```python
from build123d import *

# Parameters (mm, degrees)
SKETCH1_W           = 50.8
SKETCH1_H           = 82.55
BOSS_EXTRUDE1_DEPTH = 12.7
CUT_EXTRUDE1_DEPTH  = 1.27
SKETCH3_W           = 2.998982734
SKETCH3_H           = 7.14554636
SKETCH3_W_2         = 3.079931229
BOSS_EXTRUDE2_DEPTH = 12.7


with BuildPart() as part:
    # Sketch1 → Boss-Extrude1 (new body)
    with BuildSketch(Plane(origin=(0, 0, 0), x_dir=(1, 0, 0), z_dir=(0, 1, 0))):
        Rectangle(SKETCH1_W, SKETCH1_H)
    extrude(amount=BOSS_EXTRUDE1_DEPTH)

    # Sketch2 → Cut-Extrude1 (cut)
    with BuildSketch(Plane(origin=(0, 12.7, 0), x_dir=(1, 0, 0), z_dir=(0, 1, 0))):
        Polygon((-1.861676083, 3.013416612), (-0.314881211, 3.013416612), (-0.314881211, 2.687775586), (-1.576740185, 2.687775586), (-1.576740185, 1.710852509), (-0.314881211, 1.710852509), (-0.314881211, 1.385211483), (-1.576740185, 1.385211483), (-1.576740185, -0.161583388), (-1.861676083, -0.161583388), align=None)
        with BuildLine():
            Line((3.185759815, 2.430824464), (2.936440905, 2.240019176))
            add(Edge.make_bspline(
                [(2.936440905, 2.240019176), (2.918655563, 2.261215448), (2.883324665, 2.303322222), (2.826483817, 2.36244938), (2.767245898, 2.417844296), (2.705633552, 2.469770858), (2.64053778, 2.51641321), (2.573535484, 2.560201996), (2.503505828, 2.599452015), (2.406666755, 2.647043439), (2.279986207, 2.696706022), (2.120515174, 2.73834681), (1.954044392, 2.764854591), (1.840472284, 2.767725555), (1.782704927, 2.769185842)],
                knots=[0, 0, 0, 0, 0.757959112, 1.505699292, 2.245454638, 2.979532153, 3.711538275, 4.438200793, 5.171680507, 5.909471876, 7.393775596, 8.890124382, 10.418191784, 12, 12, 12, 12], degree=3))
            add(Edge.make_bspline(
                [(1.782704927, 2.769185842), (1.750879363, 2.768819391), (1.687523605, 2.768089888), (1.593499633, 2.758465896), (1.501231365, 2.744939298), (1.410778821, 2.724868469), (1.322257137, 2.699493308), (1.235087601, 2.669171682), (1.150532271, 2.631656935), (1.06742144, 2.590193013), (0.987793156, 2.543359546), (0.912450363, 2.492275291), (0.841667849, 2.437511896), (0.775389622, 2.378864107), (0.713547926, 2.316596042), (0.656590866, 2.250044104), (0.604715529, 2.179421061), (0.556893657, 2.105658184), (0.514064963, 2.02897033), (0.478205715, 1.949073659), (0.446451069, 1.867336366), (0.421323898, 1.782834956), (0.40143523, 1.696164018), (0.387712278, 1.607090946), (0.378197736, 1.515801822), (0.377471861, 1.453926232), (0.377105969, 1.422736523)],
                knots=[0, 0, 0, 0, 1.054917814, 2.100044995, 3.131103042, 4.146048494, 5.169673617, 6.183595914, 7.203665975, 8.234915748, 9.262203917, 10.264457458, 11.251630812, 12.227803204, 13.197192746, 14.159520551, 15.12972552, 16.100847026, 17.073214652, 18.039054194, 19.002613845, 19.979014051, 20.95965708, 21.949030935, 22.966165397, 24, 24, 24, 24], degree=3))
            add(Edge.make_bspline(
                [(0.377105969, 1.422736523), (0.378250619, 1.375808826), (0.380497988, 1.283672517), (0.400498976, 1.14871632), (0.430892881, 1.019429709), (0.476445582, 0.896620852), (0.532615007, 0.778775413), (0.603590419, 0.66788731), (0.685792563, 0.562280855), (0.780384358, 0.464451896), (0.884166777, 0.375085873), (0.995516668, 0.296390703), (1.114156701, 0.230790774), (1.23877693, 0.176202594), (1.370336333, 0.134241134), (1.508598332, 0.104700822), (1.653262214, 0.085431129), (1.752113026, 0.083586284), (1.802421474, 0.082647381)],
                knots=[0, 0, 0, 0, 1.029171465, 2.020641659, 2.987623507, 3.938342917, 4.889210282, 5.84687017, 6.821220943, 7.821438502, 8.827599549, 9.822697543, 10.807740252, 11.797342354, 12.80366471, 13.83203677, 14.896651826, 16, 16, 16, 16], degree=3))
            add(Edge.make_bspline(
                [(1.802421474, 0.082647381), (1.857850341, 0.084179345), (1.966947613, 0.087194618), (2.126938608, 0.11273908), (2.280096767, 0.154157334), (2.426430328, 0.212121877), (2.565526757, 0.28747396), (2.697603727, 0.37882132), (2.822772723, 0.487032879), (2.89803953, 0.569658288), (2.936440905, 0.611814047)],
                knots=[0, 0, 0, 0, 1.028121516, 2.023589091, 2.998037872, 3.967518031, 4.937445131, 5.927275754, 6.942489185, 8, 8, 8, 8], degree=3))
            Line((2.936440905, 0.611814047), (3.185759815, 0.422916812))
            add(Edge.make_bspline(
                [(3.185759815, 0.422916812), (3.16569553, 0.397028359), (3.125663066, 0.345375458), (3.060840436, 0.27255755), (2.992553173, 0.204064603), (2.920294065, 0.140448832), (2.844894354, 0.080437281), (2.765000185, 0.025734906), (2.681661848, -0.024421825), (2.595161714, -0.070347678), (2.505591686, -0.111094038), (2.413059092, -0.145977098), (2.317962784, -0.176026105), (2.220298416, -0.200747505), (2.119863408, -0.220043417), (2.017020192, -0.232942693), (1.911546805, -0.241780001), (1.84038923, -0.242585468), (1.804329526, -0.242993645)],
                knots=[0, 0, 0, 0, 0.986787822, 1.968848986, 2.935600012, 3.899624008, 4.868462664, 5.837806735, 6.815139263, 7.798259679, 8.787526145, 9.778297419, 10.776456485, 11.791383307, 12.812564526, 13.85620153, 14.913611965, 16, 16, 16, 16], degree=3))
            add(Edge.make_bspline(
                [(1.804329526, -0.242993645), (1.770181343, -0.24275598), (1.702657538, -0.242286028), (1.602963671, -0.234673133), (1.505908837, -0.224286586), (1.411770426, -0.208647324), (1.32003472, -0.190192101), (1.231533333, -0.165453176), (1.145395392, -0.137740717), (1.061966969, -0.105169765), (0.981177098, -0.0684158), (0.903286355, -0.026876314), (0.828330563, 0.019099377), (0.755572788, 0.068497851), (0.686087837, 0.122905832), (0.619273568, 0.181567708), (0.554755321, 0.24428576), (0.5148386, 0.289511234), (0.49476923, 0.312249745)],
                knots=[0, 0, 0, 0, 1.114604814, 2.203992996, 3.262667896, 4.300477797, 5.318619304, 6.316056647, 7.298880507, 8.271930387, 9.238335007, 10.195173496, 11.151986948, 12.108099108, 13.064862484, 14.031167946, 15.010108607, 16, 16, 16, 16], degree=3))
            add(Edge.make_bspline(
                [(0.49476923, 0.312249745), (0.462624039, 0.351747823), (0.398721742, 0.430267125), (0.316964872, 0.557526551), (0.246981019, 0.69039414), (0.190397148, 0.829567933), (0.146162382, 0.974735634), (0.115518013, 1.125970422), (0.095604771, 1.283131055), (0.093327581, 1.390025856), (0.092170071, 1.444361123)],
                knots=[0, 0, 0, 0, 0.994628077, 1.977248131, 2.950237994, 3.925870899, 4.908910175, 5.911660606, 6.938484602, 8, 8, 8, 8], degree=3))
            add(Edge.make_bspline(
                [(0.092170071, 1.444361123), (0.093580854, 1.501470713), (0.096356481, 1.613830266), (0.119938381, 1.778725209), (0.157874003, 1.936705407), (0.211755467, 2.087475946), (0.280068178, 2.231829843), (0.364456606, 2.368664365), (0.463940371, 2.498854605), (0.577739236, 2.620425129), (0.702532462, 2.731585828), (0.836171672, 2.829381455), (0.978395295, 2.910768059), (1.127636489, 2.978800292), (1.285012786, 3.031092055), (1.450188413, 3.06769816), (1.622853, 3.090482973), (1.740656772, 3.09336334), (1.800513421, 3.094826868)],
                knots=[0, 0, 0, 0, 1.032925535, 2.032216505, 3.007276963, 3.968222605, 4.92396291, 5.891752235, 6.871517503, 7.883894988, 8.900124299, 9.891468569, 10.874487609, 11.85992873, 12.854644235, 13.869047385, 14.917252991, 16, 16, 16, 16], degree=3))
            add(Edge.make_bspline(
                [(1.800513421, 3.094826868), (1.836993692, 3.0943895), (1.909202714, 3.093523773), (2.016021192, 3.085081773), (2.12001816, 3.071008716), (2.221265265, 3.051853424), (2.320255067, 3.02807964), (2.416231, 2.997109512), (2.509756237, 2.961697801), (2.600240932, 2.92091405), (2.687250946, 2.875133506), (2.770759177, 2.824863619), (2.850102299, 2.77016671), (2.925838612, 2.711507972), (2.996701175, 2.647646422), (3.064701944, 2.580338603), (3.127531637, 2.507645776), (3.166314892, 2.456478444), (3.185759815, 2.430824464)],
                knots=[0, 0, 0, 0, 1.096760587, 2.17092713, 3.219439832, 4.250915756, 5.268269357, 6.278326846, 7.281116186, 8.274029601, 9.260640565, 10.235837813, 11.203064059, 12.156899882, 13.114053108, 14.069676657, 15.032185724, 16, 16, 16, 16], degree=3))
        make_face()
    extrude(amount=-CUT_EXTRUDE1_DEPTH, mode=Mode.SUBTRACT)

    # Sketch3 → Boss-Extrude2 (add)
    with BuildSketch(Plane.XY.offset(41.275)):
        with Locations((20.244451429, 6.168632911)):
            Rectangle(SKETCH3_W, SKETCH3_H)
        with Locations((15.24371534, 6.168632911)):
            Rectangle(SKETCH3_W_2, SKETCH3_H)
    extrude(amount=BOSS_EXTRUDE2_DEPTH)


solid = part.part
```
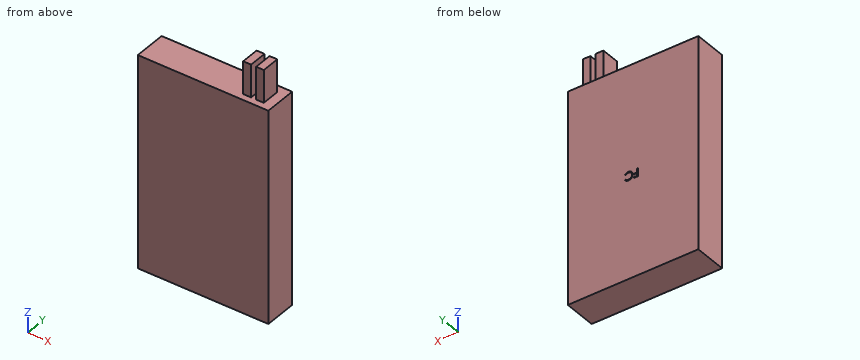
The model under review builds one solid part; all positions refer to its coordinate system, in mm. Coordinates: 2 decimals unless noted, no trailing zeros. Loops run counter-clockwise (first coordinate to the right, second up) from the corner with the lowest first, then second, coordinate; pieces in that order, holes last. Notation, with made-up numbers: (77.5, 57) -> (101.5, 57) arc R20 cw to (101.5, 74) -> close; hole circle Ø5 at (75.5, 81.5). An arc over 180 degrees is marked (long way). Answer as CSV lines item,"result".
Item 1: Take a section at B-B, the plane x = 6. State the section outline as (y, z) points (3 decimals), and give its area (3 significant figures).
Results below:
outline,"(0, -41.275) -> (12.7, -41.275) -> (12.7, 41.275) -> (0, 41.275) -> close"
area,"1,050 mm2"
Item 2: Take a section at A-A, the plane y = 7. State the section outline as (x, z) points (3 decimals), and give its area (3 significant figures).
Results below:
outline,"(-25.4, -41.275) -> (25.4, -41.275) -> (25.4, 41.275) -> (21.744, 41.275) -> (21.744, 53.975) -> (18.745, 53.975) -> (18.745, 41.275) -> (16.784, 41.275) -> (16.784, 53.975) -> (13.704, 53.975) -> (13.704, 41.275) -> (-25.4, 41.275) -> close"
area,"4,270 mm2"
Item 3: Insertion check: pin 1 (1.5 mm diameter, centred on x = -14, y = 10.5, fed in from +Z) (3 decimals); pin 2 (0.5 mm diameter, centred on x = -1.5, z = -1.5, fed in from +Y); pin 3 (2 mm diameter, centred on y = 7.5, z = 48, fed in from -X); pin 4 (2.5 mm diameter, centred on x = 20, z = 46, fed in from +Y). Each pin has a flat end and moves straight along its axis. Give the tip position at first contact, or say it passes through.
Results below:
pin 1,"stops at z = 41.275"
pin 2,"stops at y = 12.7"
pin 3,"stops at x = 13.7"
pin 4,"stops at y = 9.74"
Item 4: For L1, parallel to X at y = 6.5, z = 45.5; L2, parallel to Z at x = 5, y = 1.5 (3 decimals), list the stretches that pass through material, from the lowest coordinate up.
Results below:
L1,"x = 13.7 to 16.78, 18.74 to 21.74"
L2,"z = -41.275 to 41.275"
